from build123d import *

# Parameters (mm, degrees)
F0_R     = 2.737036
F0_R_2   = 2.5
F1_DEPTH = 6.5


with BuildPart() as f1:
    # F0 (on Top) → F1 (new body)
    with BuildSketch(Plane.XY):
        Polygon((40, 0), (-40, 0), (-40, -20), (-30, -20), (-19.393398, -30.606602), (-19.393398, -50.606602), (19.393398, -50.606602), (19.393398, -30.606602), (30, -20), (40, -20), align=None)
        with Locations((0, -27.606602)):
            Circle(F0_R, mode=Mode.SUBTRACT)
        with Locations((-32, -10)):
            Circle(F0_R_2, mode=Mode.SUBTRACT)
        with Locations((32, -10)):
            Circle(F0_R_2, mode=Mode.SUBTRACT)
    extrude(amount=F1_DEPTH)


solid = f1.part
Build history of the part. All positions in model axes, mm. A direction names the side the tool comes from. Round coordinates to 2 decimals unless told otherwise and drop trailing zeros. Loops run counter-clockwise (first coordinate to the right, second up) from the corner with the lowest first, then second, coordinate; pieces in that order, holes last. Notation, with made-up numbers: (33.25, 57.5) -> (57.25, 57.5) arc R31 ccw to (57.25, 81.5) -> close; hole circle Ø10 at (66, -13.75). An arc over 180 degrees is marked (long way). Use CSV: the item, a comma, the result in double quotes. Start each with the question number.
Q1. Saw through at D-D on x = 23. Give the cut face in (y, z), and give its area (4 significant figures).
Q2. Which spindle directions (+Z, -Z, +X, -X, +Y, -Y) get a long thin tool onto all of the face, cutting with end or side? Do faces 1 (the face through (0, -50.607, 3)), 2 (the face through (-19.393, -40, 3)), 3 (the face through (19.393, -41, 3)). Say none if no direction does.
Q3. Flat gauge pins, fed straight in: pin 1 Ø3 at (y, z) = (-45.5, 4.5) entering from -X; pin 2 Ø1.5 at (x, z) = (22.5, 3.5) entering from -Y; pin 3 Ø2 at (x, z) = (35, 2) entering from -Y. Where does each tip first touch, or does it go through?
Q4. Saw through at A-A on y = -10. Give the cut face in (x, z), and give its area (3 significant figures).
Q5. Saw through at C-C on z = 5.5. Give the cut face in (x, y).
Q6. Drill centre lines: L1, parallel to Y at x = 32, z = 4.75; L2, parallel to Y at x = 0, z = 3.75; L3, parallel to X at y = -33, z = 5.5. Where is each one in solid material? Low to high.
Q7. Saw through at B-B on x = 32. Give the cut face in (y, z), and give its area (3 significant figures).
Solutions:
1,outline,"(-27, 0) -> (0, 0) -> (0, 6.5) -> (-27, 6.5) -> close"
1,area,"175.5 mm^2"
2,face 1,"+Z, -Z, +X, -X, -Y"
2,face 2,"+Z, -Z, -X, -Y"
2,face 3,"+Z, -Z, +X, -Y"
3,pin 1,"stops at x = -19.39"
3,pin 2,"stops at y = -28.25"
3,pin 3,"stops at y = -20"
4,outline,"(-40, 0) -> (-34.5, 0) -> (-34.5, 6.5) -> (-40, 6.5) -> close; (-29.5, 0) -> (29.5, 0) -> (29.5, 6.5) -> (-29.5, 6.5) -> close; (34.5, 0) -> (40, 0) -> (40, 6.5) -> (34.5, 6.5) -> close"
4,area,"455 mm^2"
5,outline,"(-40, -20) -> (-30, -20) -> (-19.39, -30.61) -> (-19.39, -50.61) -> (19.39, -50.61) -> (19.39, -30.61) -> (30, -20) -> (40, -20) -> (40, 0) -> (-40, 0) -> close; hole circle Ø5 at (-32, -10); hole circle Ø5.47 at (0, -27.61); hole circle Ø5 at (32, -10)"
6,L1,"y = -20 to -12.5, -7.5 to 0"
6,L2,"y = -50.61 to -30.34, -24.87 to 0"
6,L3,"x = -19.39 to 19.39"
7,outline,"(-20, 0) -> (-12.5, 0) -> (-12.5, 6.5) -> (-20, 6.5) -> close; (-7.5, 0) -> (0, 0) -> (0, 6.5) -> (-7.5, 6.5) -> close"
7,area,"97.5 mm^2"
